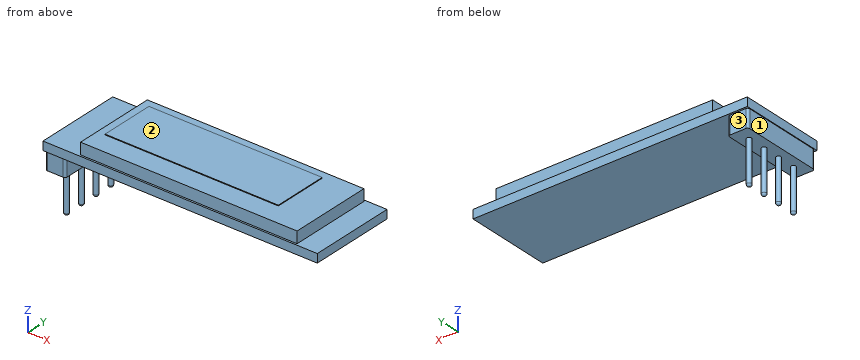
```python
from build123d import *

# Parameters (mm, degrees)
SKETCH1_W           = 38
SKETCH1_H           = 12
BOSS_EXTRUDE1_DEPTH = 1.2
SKETCH2_W           = 30
SKETCH2_H           = 11.5
BOSS_EXTRUDE2_DEPTH = 1.6
SKETCH6_W           = 2.8
SKETCH6_H           = 11.5
BOSS_EXTRUDE4_DEPTH = 2.5
SKETCH5_R           = 0.32
BOSS_EXTRUDE5_DEPTH = 8.5
FILLET1_R           = 0.3
FILLET2_R           = 0.3
SKETCH4_W           = 24
SKETCH4_H           = 7.54
BOSS_EXTRUDE6_DEPTH = 0.1


with BuildPart() as part:
    # Sketch1 → Boss-Extrude1 (new body)
    with BuildSketch(Plane.XY):
        Rectangle(SKETCH1_W, SKETCH1_H)
    extrude(amount=BOSS_EXTRUDE1_DEPTH)

    # Sketch2 → Boss-Extrude2 (add)
    with BuildSketch(Plane.XY.offset(1.2)):
        with Locations((1, 0)):
            Rectangle(SKETCH2_W, SKETCH2_H)
    extrude(amount=BOSS_EXTRUDE2_DEPTH)

    # Sketch6 → Boss-Extrude4 (add)
    with BuildSketch(Plane(origin=(0, 0, 0), x_dir=(-1, 0, 0), z_dir=(0, 0, -1))):
        with Locations((17.5, 0)):
            Rectangle(SKETCH6_W, SKETCH6_H)
    extrude(amount=BOSS_EXTRUDE4_DEPTH)

    # Sketch5 → Boss-Extrude5 (add)
    with BuildSketch(Plane(origin=(0, 0, 0), x_dir=(-1, 0, 0), z_dir=(0, 0, -1))):
        with Locations((17.5, 3.81)):
            Circle(SKETCH5_R)
        with Locations((17.5, 1.25)):
            Circle(SKETCH5_R)
        with Locations((17.5, -1.25)):
            Circle(SKETCH5_R)
        with Locations((17.5, -3.81)):
            Circle(SKETCH5_R)
    extrude(amount=BOSS_EXTRUDE5_DEPTH)

    # Fillet1
    fillet1_edges = [part.edges().sort_by_distance(p)[0] for p in [
        (-17.18, 3.81, -8.5),
        (-17.18, 1.25, -8.5),
        (-17.18, -1.25, -8.5),
        (-17.18, -3.81, -8.5),
    ]]
    fillet(fillet1_edges, radius=FILLET1_R)

    # Fillet2
    fillet2_edges = [part.edges().sort_by_distance(p)[0] for p in [
        (-16.1, 5.75, -1.25),
        (-16.1, -5.75, -1.25),
        (-18.9, -5.75, -1.25),
        (-18.9, 5.75, -1.25),
    ]]
    fillet(fillet2_edges, radius=FILLET2_R)

    # Sketch4 → Boss-Extrude6 (add)
    with BuildSketch(Plane.XY.offset(2.8)):
        with Locations((-0.9, 0.88)):
            Rectangle(SKETCH4_W, SKETCH4_H)
    extrude(amount=BOSS_EXTRUDE6_DEPTH)


solid = part.part
```
For this review, take the finished solid that the model builds, in its own axes (mm). Face numbers are marked on the shaded views. A direction names the side the tool comes from. Coordinates: 2 decimals unless noted, no trailing zeros. Write each loop counter-clockwise with the first axis right and the second up, starting at its lowest first coordinate (ties: lowest second). Pieces come first, ordered by that corner, then holes. Notation, with made-up numbers: (79.25, 14.5) - (107.25, 14.5) arc R23 ccw to (107.25, 27.5) - close; hole circle Ø10 at (-34, 75). An arc over 180 degrees is marked (long way). Answer in a Markdown table with one row per item. Add a question column.
Q1. We need section D-D, the plane z = -4.25. State the section outline as (x, y) points, and give its area (3 significant figures).
Q2. We need section B-B, the plane z = -1.25. State the section outline as (x, y) points, and give its area (3 significant figures).
Q3. For P1, Ø0.7, axis at x = -17.5, z = -1, coming from the +Y side; P2, Ø5, axis at y = -4.5, z = -7, coming from the -X side; P3, Ø6, axis at x = 6, y = 0, coming from the -Z side, all flat-tipped, find the tip position at first contact; note any pin that passes through.
Q4. For probe 1 along Z at (x, y) = (17.5, 0.75); probe 2 along X at (y, z) = (3.25, 2.75); probe 3 along Z at (x, y) = (1.5, -0.5), list the stretches that pass through material, from the lowest coordinate up.
Q5. Tool access review of the marked faces 1, 2 and 3: name each direction out of +Z, -Z, +X, -X, +Y, -Y from which nothing blocks a thin tool from reaching the whole face with its end or side.
Q6. We need section C-C, the plane y = -2.5. State the section outline as (x, z) points.
Q7. We need section A-A, the plane x = 2.5. State the section outline as (y, z) points.
Answer list:
| question | item | result |
|---|---|---|
| 1 | outline | circle Ø0.64 at (-17.5, -3.81); circle Ø0.64 at (-17.5, -1.25); circle Ø0.64 at (-17.5, 1.25); circle Ø0.64 at (-17.5, 3.81) |
| 1 | area | 1.29 mm2 |
| 2 | outline | (-18.9, -5.45) arc R0.3 ccw to (-18.6, -5.75) - (-16.4, -5.75) arc R0.3 ccw to (-16.1, -5.45) - (-16.1, 5.45) arc R0.3 ccw to (-16.4, 5.75) - (-18.6, 5.75) arc R0.3 ccw to (-18.9, 5.45) - close |
| 2 | area | 32.1 mm2 |
| 3 | P1 | stops at y = 5.75 |
| 3 | P2 | stops at x = -17.82 |
| 3 | P3 | stops at z = 0 |
| 4 | probe 1 | z = 0 to 1.2 |
| 4 | probe 2 | x = -14 to 16 |
| 4 | probe 3 | z = 0 to 2.9 |
| 5 | face 1 | -Z, -X, +Y, -Y |
| 5 | face 2 | +Z, +X, -X, +Y, -Y |
| 5 | face 3 | -Z, +X, -X, +Y |
| 6 | outline | (-19, 0) - (-18.9, 0) - (-18.9, -2.5) - (-16.1, -2.5) - (-16.1, 0) - (19, 0) - (19, 1.2) - (16, 1.2) - (16, 2.8) - (11.1, 2.8) - (11.1, 2.9) - (-12.9, 2.9) - (-12.9, 2.8) - (-14, 2.8) - (-14, 1.2) - (-19, 1.2) - close |
| 7 | outline | (-6, 0) - (6, 0) - (6, 1.2) - (5.75, 1.2) - (5.75, 2.8) - (4.65, 2.8) - (4.65, 2.9) - (-2.89, 2.9) - (-2.89, 2.8) - (-5.75, 2.8) - (-5.75, 1.2) - (-6, 1.2) - close |
